```python
from build123d import *

# Parameters (mm, degrees)
CROQUIS1_W              = 50
CROQUIS1_H              = 50
CROQUIS1_R              = 2
SALIENTE_EXTRUIR2_DEPTH = 0.8
CROQUIS4_R              = 4
CROQUIS4_W              = 3.55
CROQUIS4_H              = 40
CORTAR_EXTRUIR1_DEPTH   = 10
CORTAR_EXTRUIR2_START   = -39.374993
CROQUIS7_R              = 2
CORTAR_EXTRUIR2_DEPTH   = 28.749989
CROQUIS8_R              = 3
SALIENTE_EXTRUIR3_DEPTH = 15


with BuildPart() as part:
    # Croquis1 → Saliente-Extruir2 (new body)
    with BuildSketch(Plane.XY):
        Rectangle(CROQUIS1_W, CROQUIS1_H)
        Circle(CROQUIS1_R, mode=Mode.SUBTRACT)
    extrude(amount=SALIENTE_EXTRUIR2_DEPTH)

    # Croquis2 → Revolución1 (revolve)
    with BuildSketch(Plane(origin=(0, 0, 0), x_dir=(0, 0, -1), z_dir=(1, 0, 0))):
        Polygon((-0.8, 0), (-10.8, 0), (-10.8, 10), (-2.8, 15), (-0.8, 15), align=None)
    revolve(axis=Axis((0, 0, 0.8), (0, 0, 1)))

    # Croquis4 → Cortar-Extruir1 (cut)
    with BuildSketch(Plane.XY.offset(10.8)):
        Circle(CROQUIS4_R)
        with Locations((-6.675, 0)):
            Rectangle(CROQUIS4_W, CROQUIS4_H)
        with Locations((6.675, 0)):
            Rectangle(CROQUIS4_W, CROQUIS4_H)
    extrude(amount=-CORTAR_EXTRUIR1_DEPTH, mode=Mode.SUBTRACT)

    # Croquis7 → Cortar-Extruir2 (cut)
    with BuildSketch(Plane.ZY.offset(25).offset(CORTAR_EXTRUIR2_START)):
        with Locations((5.8, 0)):
            Circle(CROQUIS7_R)
    extrude(amount=CORTAR_EXTRUIR2_DEPTH, mode=Mode.SUBTRACT)

    # Croquis8 → Saliente-Extruir3 (add)
    with BuildSketch(Plane.XY.offset(0.8)):
        with Locations((19.8, -19.8)):
            Circle(CROQUIS8_R)
    extrude(amount=SALIENTE_EXTRUIR3_DEPTH)


solid = part.part
```
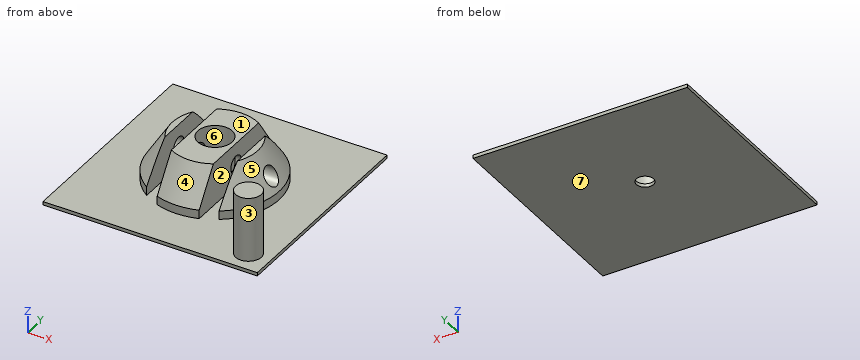
Input: part model. Units: mm. Frame: model coordinates. Face numbers are marked on the shaded views. A direction names the side the tool comes from. Coordinates: 2 decimals unless noted, no trailing zeros. Loops run counter-clockwise (first coordinate to the right, second up) from the corner with the lowest first, then second, coordinate; pieces in that order, holes last. Notation, with made-up numbers: (82, 7.5) - (104, 7.5) arc R28 cw to (104, 36.5) - close; hole circle Ø10 at (18.25, -39.75). An arc over 180 degrees is marked (long way). Answer in a Markdown table with one row per item.
(1) Cut plane B-B on z = 5.5. Count the separate pieces of the cut face and the enclosed holes in it, plus the area to 3 significant figures.
Model answer:
| item | result |
|---|---|
| separate pieces | 7 |
| enclosed holes | 0 |
| area | 326 mm² |
(2) Cut plane C-C on y = -19.8. Output: boundary loops of the cut face in (x, z).
Model answer:
| item | result |
|---|---|
| outline | (-25, 0) - (25, 0) - (25, 0.8) - (22.8, 0.8) - (22.8, 15.8) - (16.8, 15.8) - (16.8, 0.8) - (-25, 0.8) - close |
(3) Cut plane A-A on x = 0. Output: boundary loops of the cut face in (y, z), plus the area to 3 significant figures.
Model answer:
| item | result |
|---|---|
| outline | (-25, 0) - (-2, 0) - (-2, 0.8) - (-4, 0.8) - (-4, 10.8) - (-10, 10.8) - (-15, 2.8) - (-15, 0.8) - (-25, 0.8) - close; (2, 0) - (25, 0) - (25, 0.8) - (15, 0.8) - (15, 2.8) - (10, 10.8) - (4, 10.8) - (4, 0.8) - (2, 0.8) - close |
| area | 217 mm² |
(4) Cut plane D-D on x = 19.8. Output: boundary loops of the cut face in (y, z), plus the area to 3 significant figures.
Model answer:
| item | result |
|---|---|
| outline | (-25, 0) - (25, 0) - (25, 0.8) - (-16.8, 0.8) - (-16.8, 15.8) - (-22.8, 15.8) - (-22.8, 0.8) - (-25, 0.8) - close |
| area | 130 mm² |
(5) Set-up query: the marked faces 1, 2 and 3. Return all of +Z, -Z, +X, -X, +Y, -Y with unobstructed straight access to the full face (end or side cutting, diameter ignored); none if empty.
Model answer:
| item | result |
|---|---|
| face 1 | +Z, +X, -X, +Y, -Y |
| face 2 | +Z, +Y, -Y |
| face 3 | +Z |
(6) Pin query (flat end, axial travel): P1, Ø1, axis at x = 5, y = 16, coming from the +Z side; P2, Ø6.5, axis at x = -2, y = -0.5, coming from the +Z side; P3, Ø3, axis at y = 0, z = 5.8, coming from the +X side; P4, Ø5, axis at y = 0, z = 7, coming from the +X side. Return the tip coordinate at first contact, or that it passes through.
Model answer:
| item | result |
|---|---|
| P1 | stops at z = 0.8 |
| P2 | stops at z = 10.8 |
| P3 | passes through |
| P4 | stops at x = 13.19 |
(7) Mould query, pull axis X, two halves, no side actions, for the marked faces 4, 5, 6 and 7. Classes: pulls with the +X half, pulls with the -X half, needs draft (parallel to the pull), parting line crosses it, or undercut.
Model answer:
| item | result |
|---|---|
| face 4 | parting line crosses it |
| face 5 | pulls with the +X half |
| face 6 | undercut |
| face 7 | needs draft |
(8) Material intervals for L1, parallel to X at y = 3.5, z = 2.5; L2, parallel to X at y = -3.5, z = 8.25; L3, parallel to Y at x = 0, z = 0.5, sorted ascending. Write a range as from..to.
Model answer:
| item | result |
|---|---|
| L1 | x = -14.59..-8.45, -4.9..-1.94, 1.94..4.9, 8.45..14.59 |
| L2 | x = -11.05..-8.45, -4.9..-1.94, 1.94..4.9, 8.45..11.05 |
| L3 | y = -25..-2, 2..25 |
